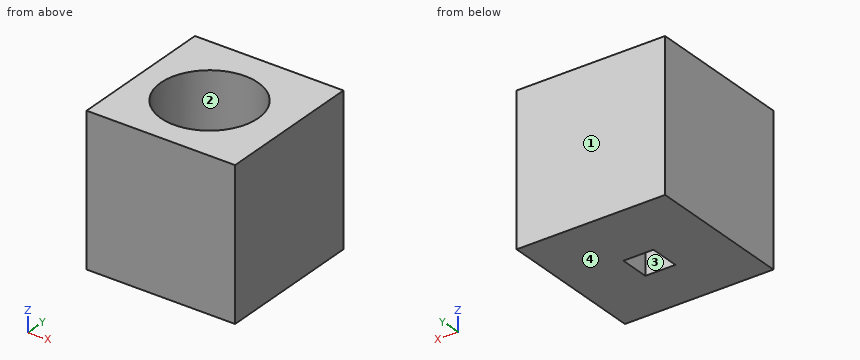
```python
from build123d import *

# Parameters (mm, degrees)
F0_R     = 16.635209
F0_W     = 10.285949
F0_H     = 10.285953
F1_DEPTH = 25.4
F0_W_2   = 50.8
F0_H_2   = 50.8
F2_DEPTH = 50.8


with BuildPart() as f1:
    # F0 (on Top) → F1 (new body)
    with BuildSketch(Plane.XY):
        with Locations((24.140496, 24.560331)):
            Circle(F0_R)
        with Locations((25.504959, 23.19587)):
            Rectangle(F0_W, F0_H, mode=Mode.SUBTRACT)
    extrude(amount=F1_DEPTH)

    # F0 (on Top) → F2 (join)
    with BuildSketch(Plane.XY):
        with Locations((25.4, 25.4)):
            Rectangle(F0_W_2, F0_H_2)
        with Locations((24.140496, 24.560331)):
            Circle(F0_R, mode=Mode.SUBTRACT)
    extrude(amount=F2_DEPTH)


solid = f1.part
```
Work out the finished part from the listing and answer in its coordinate system (mm). Face numbers are marked on the shaded views. Round coordinates to 2 decimals unless told otherwise and drop trailing zeros. Write each loop counter-clockwise with the first axis right and the second up, starting at its lowest first coordinate (ties: lowest second). Pieces come first, ordered by that corner, then holes. Notation, with made-up numbers: (41, -8) -> (90, -8) arc R31 cw to (90, 26) -> close; hole circle Ø4 at (53.5, 20.5). An arc over 180 degrees is marked (long way). Write each question's results on one line, items separated by ' | '.
Q1. Section C-C, the plane x = 8.5 is taken. Write down the section's boundary in (y, z).
Data:
outline: (0, 0) -> (50.8, 0) -> (50.8, 50.8) -> (30.23, 50.8) -> (30.23, 25.4) -> (18.89, 25.4) -> (18.89, 50.8) -> (0, 50.8) -> close
Q2. Straight lines are drawn through the part: line 1 along Y through (x, z) = (30, 5); line 2 along X through (y, z) = (24, 13.5); line 3 along Y through (x, z) = (24.5, 45.5). For each, find the intervals that lie inside material, in ascending order. Write a range as [from, to].
Data:
line 1: [0, 18.05], [28.34, 50.8] | line 2: [0, 20.36], [30.65, 50.8] | line 3: [0, 7.93], [41.19, 50.8]
Q3. Section B-B, the plane x = 28 is taken. Write down the section's boundary in (y, z).
Data:
outline: (0, 0) -> (18.05, 0) -> (18.05, 25.4) -> (8.38, 25.4) -> (8.38, 50.8) -> (0, 50.8) -> close; (28.34, 0) -> (50.8, 0) -> (50.8, 50.8) -> (40.74, 50.8) -> (40.74, 25.4) -> (28.34, 25.4) -> close
Q4. Section D-D, the plane z = 44 is taken. Write down the section's boundary in (x, y), then the cut area to 3 significant figures.
Data:
outline: (0, 0) -> (50.8, 0) -> (50.8, 50.8) -> (0, 50.8) -> close; hole circle Ø33.27 at (24.14, 24.56) | area: 1,710 mm^2
Q5. Section A-A, the plane z = 17 is taken. Write down the section's boundary in (x, y), then the cut area to 3 significant figures.
Data:
outline: (0, 0) -> (50.8, 0) -> (50.8, 50.8) -> (0, 50.8) -> close; hole (20.36, 18.05) -> (30.65, 18.05) -> (30.65, 28.34) -> (20.36, 28.34) -> close | area: 2,470 mm^2
Q6. Determine the mould class of the marked faces 1, 2, 3 and 4 for opening direction Y: released by +Y, released by -Y, zero draft, split by the parting line, or undercut.
Data:
face 1: released by +Y | face 2: undercut | face 3: undercut | face 4: zero draft
Q7. A flat-ended cylindrical pin translates along its axis: P1, Ø10, axis at x = 18.5, y = 27.5, coming from the +Z side. Find the tip coordinate at first contact, or state that the pin passes through.
Data:
P1: z = 25.4
